Build history of the part. All positions in model axes, mm. Face numbers are marked on the shaded views. Give positions to 0.01 mm unless a question says otherwise; leave off trailing zeros. Order: outer loops, then holes, each group sorted by start corner. A loop starts at its lowest first (then second) coordinate and runs counter-clockwise, first axis right, second up. Notation, with made-up numbers: (80.5, 48) - (95.5, 48) arc R21 ccw to (95.5, 52) - close; hole circle Ø5 at (5, -35.75). An arc over 180 degrees is marked (long way). Write each question's results on one line, items separated by ' | '. Start each with the question number.
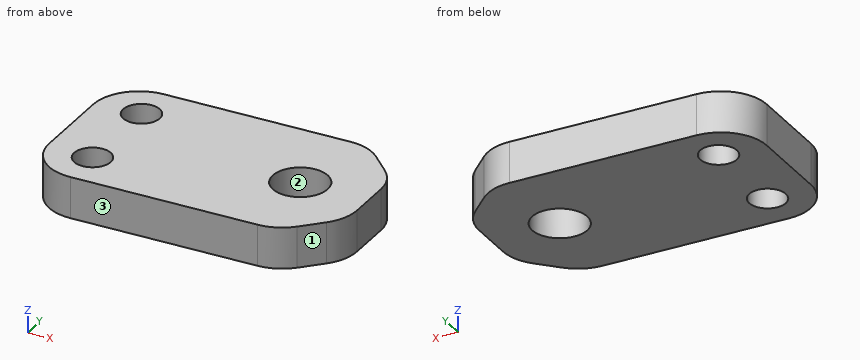
Autodesk Inventor part; units mm, degrees
ref_plane "YZ Plane" through (0, 0, 0) normal (1, 0, 0) x (0, 1, 0)
ref_plane "XZ Plane" through (0, 0, 0) normal (0, 1, 0) x (-1, 0, 0)
ref_plane "XY Plane" through (0, 0, 0) normal (0, 0, 1) x (1, 0, 0)
sketch "スケッチ2" plane through (0, 0, 0) normal (0, 0, 1) x (1, 0, 0)
  line L0 (-50, 19) -> (5, 19)
  line L1 (15, 9) -> (15, -9)
  line L2 (5, -19) -> (-50, -19)
  line L3 (-50, -19) -> (-50, 19)
  line L4 (15, 9) -> (5, 19)
  line L5 (15, -9) -> (5, -19)
  point P0 (15, -19)
  point P1 (15, 19)
  point P2 (0, 0)
  dimension "d2" = 10
  dimension "d3" = 10
  dimension "d4" = 10
  dimension "d5" = 10
  dimension "d6" = 38
  dimension "d7" = 65
  dimension "d34" = 19
  dimension "d36" = 50
extrude "押し出し2" add sketch "スケッチ2" along normal mid plane 9
sketch "スケッチ4" plane through (0, 0, -4.5) normal (0, 0, -1) x (-1, 0, 0)
  line L0 (50, 19) -> (50, -19)
  line L1 (50, -19) -> (-5, -19)
  point P0 (40, -10)
  point P1 (40, 10)
  dimension "d24" = 10
  dimension "d25" = 9
  dimension "d26" = 20
hole "穴2" at (-40, -10, -4.5) at (-40, 10, -4.5) direction (0, 0, 1) diameter 8 end through all
sketch "スケッチ5" plane through (0, 0, 4.5) normal (0, 0, 1) x (1, 0, 0)
  point P0 (0, 0)
  point P1 (0, 0)
hole "穴3" at (0, 0, 4.5) direction (0, 0, -1) diameter 12 end through all
fillet "Fillet1" radius 10 6 edges at (-50, 19, 0) (-50, -19, 0) (5, -19, 0) (15, -9, 0) (15, 9, 0) (5, 19, 0)
properties part number "210-106c" material "STEEL - HIGH GRADE ALLOY"
Item 1: Probe line 1 along Y through (x, z) = (-40, -1.25); line 2 along Y through (x, z) = (0, -1); line 3 along X through (y, z) = (0, 1). List the from-to ranges inside material, lowest first. Write a range as from..to.
Item 2: Two-plate mould, pull along X, no slides. Class the marked faces 1, 2 and 3: +X half, -X half, draft (parallel to the pull), parting line (faces both ways), or undercut.
Item 3: Cut at A-A, the plane y = 0. List the corners of the cut face in (x, z), then the cut area to 3 significant figures.
Item 4: Flat gauge pins, fed straight in: pin 1 Ø15.5 at (x, y) = (0, 0) entering from +Z; pin 2 Ø1 at (x, z) = (3.5, 0) entering from -Y; pin 3 Ø1 at (y, z) = (11, -2.5) entering from +X. Where does each tip first touch, or does it go through?
Item 5: Cut at D-D, the plane x = -42. List the corners of the cut face in (y, z).
Item 6: Cut at C-C, the plane z = -3.5. List the corners of the cut face in (x, y), then the cut area to 3 significant figures.
Item 7: Cut at B-B, the plane x = 0. List the corners of the cut face in (y, z).
Values found:
1) line 1: y = -19..-14, -6..6, 14..19 | line 2: y = -19..-6, 6..19 | line 3: x = -50..-6, 6..15
2) face 1: +X half | face 2: undercut | face 3: draft
3) outline: (-50, -4.5) - (-6, -4.5) - (-6, 4.5) - (-50, 4.5) - close; (6, -4.5) - (15, -4.5) - (15, 4.5) - (6, 4.5) - close | area: 477 mm2
4) pin 1: stops at z = 4.5 | pin 2: stops at y = -18.77 | pin 3: stops at x = 13.26
5) outline: (-18.8, -4.5) - (-13.46, -4.5) - (-13.46, 4.5) - (-18.8, 4.5) - close; (-6.54, -4.5) - (6.54, -4.5) - (6.54, 4.5) - (-6.54, 4.5) - close; (13.46, -4.5) - (18.8, -4.5) - (18.8, 4.5) - (13.46, 4.5) - close
6) outline: (-50, -9) arc R10 ccw to (-40, -19) - (0.86, -19) arc R10 ccw to (7.93, -16.07) - (12.07, -11.93) arc R10 ccw to (15, -4.86) - (15, 4.86) arc R10 ccw to (12.07, 11.93) - (7.93, 16.07) arc R10 ccw to (0.86, 19) - (-40, 19) arc R10 ccw to (-50, 9) - close; hole circle Ø8 at (-40, -10); hole circle Ø8 at (-40, 10); hole circle Ø12 at (0, 0) | area: 2,100 mm2
7) outline: (-19, -4.5) - (-6, -4.5) - (-6, 4.5) - (-19, 4.5) - close; (6, -4.5) - (19, -4.5) - (19, 4.5) - (6, 4.5) - close
